from build123d import *

# Parameters (mm, degrees)
SKETCH1_R           = 1.4
BOSS_EXTRUDE2_DEPTH = 2.2


with BuildPart() as part:
    # Sketch1 → Boss-Extrude2 (new body)
    with BuildSketch(Plane(origin=(0, 0, 0), x_dir=(1, 0, 0), z_dir=(0, 1, 0))):
        with BuildLine():
            Line((16.3, 94), (11.375, 94))
            Line((11.375, 94), (11.375, 82))
            Line((11.375, 82), (-11.375, 82))
            Line((-11.375, 82), (-11.375, 94))
            Line((-11.375, 94), (-16.3, 94))
            Line((-16.3, 94), (-16.3, -93.009457189))
            ThreePointArc((-16.3, -93.009457189), (-18.198030993, -92.065396391), (-20.256978495, -91.560908909))
            ThreePointArc((-20.256978495, -91.560908909), (-20.608541379, -92.008832104), (-20.950210791, -92.464346827))
            ThreePointArc((-20.950210791, -92.464346827), (-19.767163473, -94.547256661), (-18.105269554, -96.272429968))
            ThreePointArc((-18.105269554, -96.272429968), (-18.600034687, -97.087129259), (-19.058202403, -97.922958078))
            ThreePointArc((-19.058202403, -97.922958078), (-21.383193272, -97.34630238), (-23.778569761, -97.363208265))
            ThreePointArc((-23.778569761, -97.363208265), (-24.002222377, -97.886860017), (-24.214353801, -98.415284003))
            ThreePointArc((-24.214353801, -98.415284003), (-22.532521108, -100.121025228), (-20.480747143, -101.357284883))
            ThreePointArc((-20.480747143, -101.357284883), (-20.747793871, -102.272278608), (-20.974021483, -103.198209782))
            ThreePointArc((-20.974021483, -103.198209782), (-23.369039687, -103.242955066), (-25.678420136, -103.879253953))
            ThreePointArc((-25.678420136, -103.879253953), (-25.758920927, -104.442948261), (-25.827057957, -105.008270289))
            ThreePointArc((-25.827057957, -105.008270289), (-23.761054008, -106.220599459), (-21.459225003, -106.88369641))
            ThreePointArc((-21.459225003, -106.88369641), (-21.480354532, -107.836629259), (-21.459225003, -108.789562107))
            ThreePointArc((-21.459225003, -108.789562107), (-23.761054008, -109.452659058), (-25.827057957, -110.664988228))
            ThreePointArc((-25.827057957, -110.664988228), (-25.758920927, -111.230310256), (-25.678420136, -111.794004564))
            ThreePointArc((-25.678420136, -111.794004564), (-23.369039687, -112.430303451), (-20.974021484, -112.475048735))
            ThreePointArc((-20.974021484, -112.475048735), (-20.747793871, -113.400979909), (-20.480747144, -114.315973634))
            ThreePointArc((-20.480747144, -114.315973634), (-22.532521108, -115.552233289), (-24.214353801, -117.257974514))
            ThreePointArc((-24.214353801, -117.257974514), (-24.002222377, -117.7863985), (-23.778569761, -118.310050252))
            ThreePointArc((-23.778569761, -118.310050252), (-21.383193272, -118.326956137), (-19.058202403, -117.750300439))
            ThreePointArc((-19.058202403, -117.750300439), (-18.600034687, -118.586129259), (-18.105269555, -119.40082855))
            ThreePointArc((-18.105269555, -119.40082855), (-19.767163473, -121.126001856), (-20.950210791, -123.20891169))
            ThreePointArc((-20.950210791, -123.20891169), (-20.608541379, -123.664426413), (-20.256978495, -124.112349608))
            ThreePointArc((-20.256978495, -124.112349608), (-17.938846915, -123.508710383), (-15.842327667, -122.349951835))
            ThreePointArc((-15.842327667, -122.349951835), (-15.18344322, -123.038717947), (-14.494677108, -123.697602394))
            ThreePointArc((-14.494677108, -123.697602394), (-15.653435656, -125.794121643), (-16.257074881, -128.112253222))
            ThreePointArc((-16.257074881, -128.112253222), (-15.809151686, -128.463816106), (-15.353636963, -128.805485519))
            ThreePointArc((-15.353636963, -128.805485519), (-13.270727129, -127.6224382), (-11.545553822, -125.960544282))
            ThreePointArc((-11.545553822, -125.960544282), (-10.730854531, -126.455309415), (-9.895025712, -126.91347713))
            ThreePointArc((-9.895025712, -126.91347713), (-10.47168141, -129.238467999), (-10.454775525, -131.633844488))
            ThreePointArc((-10.454775525, -131.633844488), (-9.931123773, -131.857497104), (-9.402699787, -132.069628528))
            ThreePointArc((-9.402699787, -132.069628528), (-7.696958562, -130.387795835), (-6.460698907, -128.336021871))
            ThreePointArc((-6.460698907, -128.336021871), (-5.545705182, -128.603068598), (-4.619774008, -128.829296211))
            ThreePointArc((-4.619774008, -128.829296211), (-4.575028724, -131.224314414), (-3.938729837, -133.533694863))
            ThreePointArc((-3.938729837, -133.533694863), (-3.375035529, -133.614195654), (-2.809713501, -133.682332684))
            ThreePointArc((-2.809713501, -133.682332684), (-1.597384331, -131.616328735), (-0.93428738, -129.31449973))
            ThreePointArc((-0.93428738, -129.31449973), (0.018645469, -129.335629259), (0.971578317, -129.31449973))
            ThreePointArc((0.971578317, -129.31449973), (1.634675268, -131.616328735), (2.847004438, -133.682332684))
            ThreePointArc((2.847004438, -133.682332684), (3.412326466, -133.614195654), (3.976020774, -133.533694863))
            ThreePointArc((3.976020774, -133.533694863), (4.612319661, -131.224314414), (4.657064945, -128.829296211))
            ThreePointArc((4.657064945, -128.829296211), (5.582996119, -128.603068598), (6.497989844, -128.336021871))
            ThreePointArc((6.497989844, -128.336021871), (7.734249499, -130.387795835), (9.439990724, -132.069628528))
            ThreePointArc((9.439990724, -132.069628528), (9.96841471, -131.857497104), (10.492066462, -131.633844488))
            ThreePointArc((10.492066462, -131.633844488), (10.508972347, -129.238467999), (9.932316649, -126.91347713))
            ThreePointArc((9.932316649, -126.91347713), (10.768145469, -126.455309415), (11.582844759, -125.960544282))
            ThreePointArc((11.582844759, -125.960544282), (13.308018066, -127.6224382), (15.3909279, -128.805485518))
            ThreePointArc((15.3909279, -128.805485518), (15.846442623, -128.463816106), (16.294365818, -128.112253222))
            ThreePointArc((16.294365818, -128.112253222), (15.690726593, -125.794121643), (14.531968045, -123.697602394))
            ThreePointArc((14.531968045, -123.697602394), (15.220734157, -123.038717947), (15.879618604, -122.349951835))
            ThreePointArc((15.879618604, -122.349951835), (17.976137853, -123.508710383), (20.294269432, -124.112349608))
            ThreePointArc((20.294269432, -124.112349608), (20.645832316, -123.664426413), (20.987501728, -123.20891169))
            ThreePointArc((20.987501728, -123.20891169), (19.80445441, -121.126001856), (18.142560492, -119.400828549))
            ThreePointArc((18.142560492, -119.400828549), (18.637325625, -118.586129259), (19.09549334, -117.750300439))
            ThreePointArc((19.09549334, -117.750300439), (21.420484209, -118.326956137), (23.815860698, -118.310050252))
            ThreePointArc((23.815860698, -118.310050252), (24.039513314, -117.7863985), (24.251644738, -117.257974514))
            ThreePointArc((24.251644738, -117.257974514), (22.569812045, -115.552233289), (20.518038081, -114.315973634))
            ThreePointArc((20.518038081, -114.315973634), (20.785084808, -113.400979909), (21.011312421, -112.475048735))
            ThreePointArc((21.011312421, -112.475048735), (23.406330624, -112.430303451), (25.715711073, -111.794004564))
            ThreePointArc((25.715711073, -111.794004564), (25.796211864, -111.230310256), (25.864348894, -110.664988228))
            ThreePointArc((25.864348894, -110.664988228), (23.798344945, -109.452659058), (21.49651594, -108.789562107))
            ThreePointArc((21.49651594, -108.789562107), (21.517645469, -107.836629259), (21.49651594, -106.88369641))
            ThreePointArc((21.49651594, -106.88369641), (23.798344945, -106.220599459), (25.864348894, -105.008270289))
            ThreePointArc((25.864348894, -105.008270289), (25.796211864, -104.442948261), (25.715711073, -103.879253953))
            ThreePointArc((25.715711073, -103.879253953), (23.406330624, -103.242955066), (21.011312421, -103.198209782))
            ThreePointArc((21.011312421, -103.198209782), (20.785084808, -102.272278608), (20.518038081, -101.357284883))
            ThreePointArc((20.518038081, -101.357284883), (22.569812045, -100.121025228), (24.251644738, -98.415284003))
            ThreePointArc((24.251644738, -98.415284003), (24.039513314, -97.886860017), (23.815860698, -97.363208265))
            ThreePointArc((23.815860698, -97.363208265), (21.420484209, -97.34630238), (19.09549334, -97.922958078))
            ThreePointArc((19.09549334, -97.922958078), (18.637325625, -97.087129259), (18.142560492, -96.272429968))
            ThreePointArc((18.142560492, -96.272429968), (19.80445441, -94.547256661), (20.987501728, -92.464346827))
            ThreePointArc((20.987501728, -92.464346827), (20.645832316, -92.008832104), (20.294269432, -91.560908909))
            ThreePointArc((20.294269432, -91.560908909), (18.214473173, -92.073055949), (16.3, -93.033597224))
            Line((16.3, -93.033597224), (16.3, 94))
        make_face()
        with Locations((0.018645469, -107.836629259)):
            Circle(SKETCH1_R, mode=Mode.SUBTRACT)
    extrude(amount=BOSS_EXTRUDE2_DEPTH)


solid = part.part
Source: CAD feature listing. Evaluate the final solid. Frame: model axes, mm. Give positions to 0.01 mm unless a question says otherwise; leave off trailing zeros. Order: outer loops, then holes, each group sorted by start corner. A loop starts at its lowest first (then second) coordinate and runs counter-clockwise, first axis right, second up. Notation, with made-up numbers: (1, 18.5) -> (11, 18.5) arc R22 cw to (11, 41.5) -> close; hole circle Ø9 at (3.25, -0.75). An arc over 180 degrees is marked (long way). Write item = value, one per line.
Q1. Cut plane A-A, the plane z = 37. Output: boundary loops of the cut face in (x, y), and give its area (3 significant figures).
Data:
outline = (-16.3, 0) -> (16.3, 0) -> (16.3, 2.2) -> (-16.3, 2.2) -> close
area = 71.7 mm^2
Q2. Material intervals for line 1 (Z direction, x = -19, y = 1.4); line 2 (Z direction, x = -22, y = 0.75); line 3 (Z direction, x = 0, y = 1.55), sorted ascending. Write a range as from..to.
Data:
line_1 = 91.81..95.45, 97.81..117.86, 120.22..123.86
line_2 = 97.29..100.51, 103.14..106.78, 108.89..112.53, 115.16..118.38
line_3 = -82..106.44, 109.24..129.34
Q3. Pin query (flat end, axial travel): pin 1 (1.1 mm diameter, centred on y = 1.5, z = -89.5, fed in from -X); pin 2 (0.7 mm diameter, centred on x = 1.5, y = 1.5, fed in from -Z). Return the tip coordinate at first contact, or that it passes through.
Data:
pin_1 = -16.3
pin_2 = -82
